Geometry: final body of the model. Coordinates: model frame, mm. Give positions to 0.01 mm unless a question says otherwise; leave off trailing zeros. Write each loop counter-clockwise with the first axis right and the second up, starting at its lowest first coordinate (ties: lowest second). Pieces come first, ordered by that corner, then holes.
from build123d import *

# Parameters (mm, degrees)
F0_R     = 37
F0_R_2   = 3.4
F0_R_3   = 25
F1_DEPTH = 1


with BuildPart() as f1:
    # F0 (on Top) → F1 (new body)
    with BuildSketch(Plane.XY):
        Circle(F0_R)
        with Locations((-9.579527, -29.482752)):
            Circle(F0_R_2, mode=Mode.SUBTRACT)
        with Locations((-18.221343, -25.079527)):
            Circle(F0_R_2, mode=Mode.SUBTRACT)
        with Locations((-29.482752, -9.579527)):
            Circle(F0_R_2, mode=Mode.SUBTRACT)
        with Locations((-25.079527, -18.221343)):
            Circle(F0_R_2, mode=Mode.SUBTRACT)
        with Locations((0, -31)):
            Circle(F0_R_2, mode=Mode.SUBTRACT)
        with Locations((9.579527, -29.482752)):
            Circle(F0_R_2, mode=Mode.SUBTRACT)
        with Locations((18.221343, -25.079527)):
            Circle(F0_R_2, mode=Mode.SUBTRACT)
        with Locations((25.079527, -18.221343)):
            Circle(F0_R_2, mode=Mode.SUBTRACT)
        with Locations((29.482752, -9.579527)):
            Circle(F0_R_2, mode=Mode.SUBTRACT)
        with Locations((-31, 0)):
            Circle(F0_R_2, mode=Mode.SUBTRACT)
        with Locations((-29.482752, 9.579527)):
            Circle(F0_R_2, mode=Mode.SUBTRACT)
        with Locations((-25.079527, 18.221343)):
            Circle(F0_R_2, mode=Mode.SUBTRACT)
        with Locations((-18.221343, 25.079527)):
            Circle(F0_R_2, mode=Mode.SUBTRACT)
        with Locations((-9.579527, 29.482752)):
            Circle(F0_R_2, mode=Mode.SUBTRACT)
        Circle(F0_R_3, mode=Mode.SUBTRACT)
        with Locations((31, 0)):
            Circle(F0_R_2, mode=Mode.SUBTRACT)
        with Locations((25.079527, 18.221343)):
            Circle(F0_R_2, mode=Mode.SUBTRACT)
        with Locations((29.482752, 9.579527)):
            Circle(F0_R_2, mode=Mode.SUBTRACT)
        with Locations((18.221343, 25.079527)):
            Circle(F0_R_2, mode=Mode.SUBTRACT)
        with Locations((0, 31)):
            Circle(F0_R_2, mode=Mode.SUBTRACT)
        with Locations((9.579527, 29.482752)):
            Circle(F0_R_2, mode=Mode.SUBTRACT)
    extrude(amount=F1_DEPTH)


solid = f1.part
Q1. Pin query (flat end, axial travel): P1, Ø5.5, axis at x = -29.48, y = -9.58, coming from the +Z side. Return the tip coordinate at first contact, or that it passes through.
Filled sheet:
P1: passes through
Q2. Pull-direction query (Y, two-part tool) for faces 1 (the flat face through (-6, 25, 0)), 2 (the cylindrical face through (-0.44, -27.63, 0.49)); classes: released by +Y, released by -Y, zero draft, split by the parting line, or undercut.
Filled sheet:
face 1: zero draft
face 2: undercut
Q3. Ray query, line 1 along X through (y, z) = (8.5, 0.9); line 2 along Y through (x, z) = (31, 0.4); line 3 along Y through (x, z) = (-22, 0.8). Return the intervals inside material, ascending.
Filled sheet:
line 1: x = -36.01 to -32.71, -26.26 to -23.51, 23.51 to 26.26, 32.71 to 36.01
line 2: y = -20.2 to -12.62, -6.54 to -3.4, 3.4 to 6.54, 12.62 to 20.2
line 3: y = -29.75 to -19.66, -16.78 to -11.87, 11.87 to 16.78, 19.66 to 29.75
Q4. Section C-C on z = 0.45. Count the separate pieces of the cut face and the enclosed holes in it, plus the area to 3 significant figures.
Filled sheet:
separate pieces: 1
enclosed holes: 21
area: 1,610 mm2
Q5. Section A-A on y = 0. Output: boundary loops of the cut face in (x, z), plus the area to 3 significant figures.
Filled sheet:
outline: (-37, 0) - (-34.4, 0) - (-34.4, 1) - (-37, 1) - close; (-27.6, 0) - (-25, 0) - (-25, 1) - (-27.6, 1) - close; (25, 0) - (27.6, 0) - (27.6, 1) - (25, 1) - close; (34.4, 0) - (37, 0) - (37, 1) - (34.4, 1) - close
area: 10.4 mm2
